Autodesk Inventor part; units mm, degrees
ref_plane "YZ Plane" through (0, 0, 0) normal (1, 0, 0) x (0, 1, 0)
ref_plane "XZ Plane" through (0, 0, 0) normal (0, 1, 0) x (-1, 0, 0)
ref_plane "XY Plane" through (0, 0, 0) normal (0, 0, 1) x (1, 0, 0)
sketch "Sketch4" plane through (0, 0, 0) normal (0, 0, 1) x (1, 0, 0)
  line L0 (10.9923, 14.2423) -> (-9.6452, 14.2423)
  line L1 (11.786, 15.036) -> (11.786, 25.9263)
  line L2 (13.3735, 26.9423) -> (11.786, 26.9423)
  line L3 (-10.439, 15.036) -> (-10.439, 25.9263)
  line L4 (-10.439, 26.9423) -> (-12.0265, 26.9423)
  arc A0 (-10.439, 15.036) -> (-9.6452, 14.2423) centre (-9.6452, 15.036) ccw
  arc A1 (10.9923, 14.2423) -> (11.786, 15.036) centre (10.9923, 15.036) ccw
  arc A2 (11.786, -24.6515) -> (10.9923, -23.8577) centre (10.9923, -24.6515) ccw
  line L5 (-9.6452, -23.8577) -> (10.9923, -23.8577)
  arc A3 (-9.6452, -23.8577) -> (-10.439, -24.6515) centre (-9.6452, -24.6515) ccw
  line L6 (-10.439, -24.6515) -> (-10.439, -36.5577)
  line L7 (11.786, -24.6515) -> (11.786, -36.5577)
  line L8 (11.786, 26.9423) -> (11.786, 25.9263)
  line L9 (-10.439, 26.9423) -> (-10.439, 25.9263)
  line L10 (11.786, -24.6515) -> (-10.439, -24.6515)
  line L11 (11.786, 15.036) -> (-10.439, 15.036)
  line L12 (11.786, 26.9423) -> (11.532, 26.9423)
  line L13 (11.532, 26.9423) -> (11.532, 15.036)
  line L14 (-10.439, 26.9423) -> (-10.185, 26.9423)
  line L15 (-10.185, 26.9423) -> (-10.185, 15.036)
  line L16 (11.532, 26.9423) -> (-10.185, 26.9423)
  line L17 (11.786, -24.6515) -> (11.532, -24.6515)
  line L18 (11.532, -24.6515) -> (11.532, -36.5577)
  line L19 (11.532, -36.5577) -> (11.786, -36.5577)
  line L20 (11.786, -36.5577) -> (11.786, -24.6515)
  line L21 (-10.439, -24.6515) -> (-10.185, -24.6515)
  line L22 (-10.185, -24.6515) -> (-10.185, -36.5577)
  line L23 (-10.185, -36.5577) -> (-10.439, -36.5577)
  line L24 (-10.439, -36.5577) -> (-10.439, -24.6515)
  line L25 (11.532, -36.5577) -> (-10.439, -36.5577)
  line L26 (0, 14.2423) -> (0, -23.8577)
  point P0 (0, 0)
  dimension "d5" = 22.225
  dimension "d6" = 0.254
  dimension "d7" = 0.254
  dimension "d14" = 38.1
extrude "Extrusion2" add sketch "Sketch4" against normal blind 25.4 contours L11 L15 L16 L13 | L18 L25 L22 L10
sketch "Sketch5" plane through (11.532, -36.5577, 0) normal (1, 0, 0) x (0, 0, -1)
  point P0 (0, 36.5577)
sketch "Sketch6" plane through (11.532, -36.5577, 0) normal (1, 0, 0) x (0, 0, -1)
  line L0 (0, 51.5938) -> (0, 63.5)
  line L1 (0, 51.5938) -> (25.4, 51.5938)
  line L2 (25.4, 63.5) -> (25.4, 51.5938)
  line L3 (0, 63.5) -> (25.4, 63.5)
  line L4 (0, 0) -> (0, 11.9062)
  line L5 (0, 0) -> (25.4, 0)
  line L6 (25.4, 11.9062) -> (25.4, 0)
  line L7 (0, 11.9062) -> (25.4, 11.9062)
  line L8 (25.4, 63.5) -> (25.4, 57.15)
  line L9 (25.4, 57.15) -> (19.05, 57.15)
  line L10 (25.4, 0) -> (25.4, 6.35)
  line L11 (25.4, 6.35) -> (19.05, 6.35)
  line L12 (25.4, 62.484) -> (25.4, 51.5938)
  line L13 (37.3758, 42.3425) -> (37.3758, 45.2438)
  line L14 (37.3758, 63.5) -> (25.4, 63.5)
  line L15 (37.3758, 0) -> (25.4, 0)
  line L16 (25.4, 63.5) -> (37.3758, 63.5)
  line L17 (46.355, 51.9072) -> (46.355, 11.5928)
  line L18 (37.3758, 0) -> (25.4, 0)
  line L19 (25.4, 51.5938) -> (31.0258, 51.5938)
  line L20 (25.4, 11.9062) -> (31.0258, 11.9062)
  arc A0 (37.3758, 45.2438) -> (31.0258, 51.5938) centre (31.0258, 45.2438) ccw
  line L21 (46.355, 51.9072) -> (46.355, 50.8)
  arc A1 (46.355, 50.8) -> (37.3758, 63.5) centre (33.6671, 51.3536) ccw
  arc A2 (31.0258, 11.9062) -> (37.3758, 18.2562) centre (31.0258, 18.2562) ccw
  line L22 (46.355, 11.5928) -> (46.355, 12.7)
  arc A3 (37.3758, 0) -> (46.355, 12.7) centre (33.6671, 12.1464) ccw
  line L23 (37.3758, 42.3425) -> (37.3758, 18.2562)
  line L24 (25.4, 6.35) -> (19.05, 6.35)
  circle A4 centre (19.05, 57.15) radius 2.3241
  circle A5 centre (6.35, 57.15) radius 2.3241
  line L25 (25.4, 6.35) -> (19.05, 6.35)
  circle A6 centre (19.05, 6.35) radius 2.3241
  line L26 (19.05, 6.35) -> (6.35, 6.35)
  circle A7 centre (6.35, 6.35) radius 2.3241
  point P0 (0, 36.5577)
  dimension "d15" = 6.35
  dimension "d16" = 6.35
  dimension "d17" = 6.35
  dimension "d35" = 4.6482
  dimension "d36" = 4.6482
  dimension "d37" = 12.7
  dimension "d38" = 4.6482
extrude "Extrusion3" add sketch "Sketch6" against normal up to surface (21.717 mm away) contours L2 L14 A1 L17 A3 L15 L6 L20 A2 L23 L13 A0 L19
extrude "Extrusion4" cut sketch "Sketch6" along normal through all both and the other way through all contours A6 L26 L11 | L11 L26 A6 | A4 | A5 | A7
fillet "Fillet1" radius 13.97 2 edges at (0.6735, 26.9423, -37.3758) (0.6735, -36.5577, -37.3758)
fillet_without_effect "Fillet2"
properties part number "Front_support"
Can you work these out from the model? Positions are in its coordinate system, mm. A direction names the side the tool comes from. Give positions to 0.01 mm unless a question says otherwise; leave off trailing zeros. Order: outer loops, then holes, each group sorted by start corner. A loop starts at its lowest first (then second) coordinate and runs counter-clockwise, first axis right, second up. Notation, with made-up numbers: M 48,45.25 L 74,45.25 A17 cw 74,63.25 Z; hole C 13.5,-4.75 d5. An arc over 180 degrees is marked long. Use one line per item in the form item = value. Start each with the question number.
Item 1: We'd pull the mould along Y, two halves only. Please class faces 1 (the cylindrical face through (0.826, 18.323, -5.846)), 2 (the cylindrical face through (0.826, 13.127, -35.565)), 3 (the flat face through (1, -5, -46.355)), 4 (the flat face through (1, 26.942, -16)): +Y half, -Y half, draft (parallel to the pull), parting line (faces both ways), or undercut.
Item 2: For faces 5 (the flat face through (1, -24.652, -15)), 6 (the cylindrical face through (0.826, -32.477, -5.846)), which set-ups out of +Z, -Z, +X, -X, +Y, -Y let a thin tool reach every point of the face, with its end or its side?
Item 3: Will these pins go through, and if not, where does the flat tip stop? pin 1 Ø12 at (x, y) = (-0.5, 14) entering from -Z (3 decimals); pin 2 Ø2 at (x, y) = (-6.5, -12.5) entering from +Z.
Item 4: If we section it at B-B (z = -6.35): Write out the boundary of the cut face in (x, y) (1 decimal), then the cut area to 3 significant figures.
Item 5: If I drill on line 1 along Y through (x, z) = (-1.5, -6.35); line 2 along Y through (x, z) = (10.75, -10.5); line 3 along Z through (x, y) = (-5.25, -3.5) (3 decimals), over which ranges is the centre line in solid material (lowest first)?
Item 6: If we section it at A-A (z = -27.5): Write out the boundary of the cut face in (x, y) (1 decimal).
Item 7: If we section it at D-D (y = -4): Write out the boundary of the cut face in (x, z) (3 decimals).
Outcome:
q1.face_1 = undercut
q1.face_2 = undercut
q1.face_3 = draft
q1.face_4 = +Y half
q2.face_5 = +Z, +X, -X
q2.face_6 = +X, -X
q3.pin_1 = -46.355
q3.pin_2 = -37.38
q4.outline = M -10.2,-36.6 L 11.5,-36.6 L 11.5,-32.5 L -10.2,-32.5 Z; M -10.2,-27.9 L 11.5,-27.9 L 11.5,-24.7 L -10.2,-24.7 Z; M -10.2,15 L 11.5,15 L 11.5,18.3 L -10.2,18.3 Z; M -10.2,22.9 L 11.5,22.9 L 11.5,26.9 L -10.2,26.9 Z
q4.area = 315 mm2
q5.line_1 = -36.56 to -32.53, -27.88 to -24.65, 15.04 to 18.27, 22.92 to 26.94
q5.line_2 = -36.56 to -24.65, 15.04 to 26.94
q5.line_3 = -46.355 to -37.376
q6.outline = M -10.2,-36.6 L 11.5,-36.6 L 11.5,-24.7 L -10.2,-24.7 Z; M -10.2,15 L 11.5,15 L 11.5,26.9 L -10.2,26.9 Z
q7.outline = M -10.185,-46.355 L 11.532,-46.355 L 11.532,-37.376 L -10.185,-37.376 Z
